Design review of the part built by this model. Coordinates are the model's own, in mm. A direction names the side the tool comes from. Round coordinates to 2 decimals unless told otherwise and drop trailing zeros. Loops run counter-clockwise (first coordinate to the right, second up) from the corner with the lowest first, then second, coordinate; pieces in that order, holes last. Notation, with made-up numbers: M -19.75,45 L 26.25,45 A30 cw 26.25,71 Z; hole C 18.5,-33 d10. An arc over 180 degrees is marked long. One line per item, written item: value. Start each with the question number.
Item 1: Clearance check with a flat-ended pin moving along its axis: pin 1 (1.3 mm diameter, centred on y = 3, z = -1, fed in from -X). State where the tip first meets the part, or that it passes through.
Item 2: We need section A-A (z = 1). Write out the cut boundary in (x, y), then the cut area to 3 significant figures.
Item 3: We need section D-D (x = 26). Write out the cut boundary in (y, z).
Item 4: For faces 1 (the flat face through (57.2, 0, -2)), 2 (the flat face through (4, -3.5, 1)), 3 (the flat face through (55.2, 0, -2)), list the 3-axis set-ups (+Z, -Z, +X, -X, +Y, -Y) from which the entire face can be reached by the end or side of a thin tool; tool diameter is ignored.
Item 5: We need section C-C (x = -33). Write out the cut boundary in (y, z), then the cut area to 3 significant figures.
Item 6: For line 1 along X through (y, z) = (-2.25, 1.25); line 2 along Z through (x, y) = (-1.5, -1.75); line 3 along Y through (x, z) = (48, -3.25), list the stretches that pass through material, from the lowest coordinate up.
Item 7: We need section B-B (y = 1.75). Write out the cut boundary in (x, z).
Item 8: Mouldability with a two-part tool opening along Z and no side actions: class faces 4 (the flat face through (0, -8.25, -2)), 5 (the flat face through (-1, 0, 0)), 6 (the flat face through (0, 0, -6.2)) as released by +Z, released by -Z, zero draft, split by the parting line, or undercut.
from build123d import *

# Parameters (mm, degrees)
F2_W     = 110.4
F2_H     = 12.5
F2_W_2   = 7
F2_H_2   = 7
F3_DEPTH = 2
F4_DEPTH = 2
F5_DEPTH = 2
F6_W     = 2
F6_H     = 4.2
F7_DEPTH = 110.4
F8_W     = 16.5
F8_H     = 8.2
F9_DEPTH = 2


with BuildPart() as f3:
    # F2 (on Top) → F3 (new body)
    with BuildSketch(Plane.XY):
        Rectangle(F2_W, F2_H)
        with Locations((-23.8, 0)):
            Rectangle(F2_W_2, F2_H_2, mode=Mode.SUBTRACT)
        with Locations((4.2, 0)):
            Rectangle(F2_W_2, F2_H_2, mode=Mode.SUBTRACT)
        with Locations((27.2, 0)):
            Rectangle(F2_W_2, F2_H_2, mode=Mode.SUBTRACT)
    extrude(amount=F3_DEPTH)

    # F4 (add): a face of the model
    f4_faces = [f3.faces().sort_by_distance(p)[0] for p in [
        (0, -6.25, 1),
    ]]
    extrude(f4_faces, amount=F4_DEPTH)

    # F5 (add): a face of the model
    f5_faces = [f3.faces().sort_by_distance(p)[0] for p in [
        (0, 6.25, 1),
    ]]
    extrude(f5_faces, amount=F5_DEPTH)

    # F6 (on face) → F7 (join)
    with BuildSketch(Plane(origin=(-55.2, 0, 0), x_dir=(0, -1, 0), z_dir=(-1, 0, 0))):
        with Locations((7.25, -2.1)):
            Rectangle(F6_W, F6_H)
        Polygon((-6.25, -4.2), (-8.25, -4.2), (-8.25, -6.2), (8.25, -6.2), (8.25, -4.2), (6.25, -4.2), align=None)
        with Locations((-7.25, -2.1)):
            Rectangle(F6_W, F6_H)
    extrude(amount=-F7_DEPTH)

    # F8 (on face) → F9 (join)
    with BuildSketch(Plane.YZ.offset(55.2)):
        with Locations((0, -2.1)):
            Rectangle(F8_W, F8_H)
    extrude(amount=F9_DEPTH)


solid = f3.part
A:
1. pin 1: x = 55.2
2. outline: M -55.2,-8.25 L 57.2,-8.25 L 57.2,8.25 L -55.2,8.25 Z; hole M -27.3,-3.5 L -20.3,-3.5 L -20.3,3.5 L -27.3,3.5 Z; hole M 0.7,-3.5 L 7.7,-3.5 L 7.7,3.5 L 0.7,3.5 Z; hole M 23.7,-3.5 L 30.7,-3.5 L 30.7,3.5 L 23.7,3.5 Z
2. area: 1,710 mm2
3. outline: M -8.25,-6.2 L 8.25,-6.2 L 8.25,2 L 3.5,2 L 3.5,0 L 6.25,0 L 6.25,-4.2 L -6.25,-4.2 L -6.25,0 L -3.5,0 L -3.5,2 L -8.25,2 Z
4. face 1: +Z, -Z, +X, +Y, -Y
4. face 2: +Z
4. face 3: -X
5. outline: M -8.25,-6.2 L 8.25,-6.2 L 8.25,2 L -8.25,2 Z; hole M -6.25,-4.2 L 6.25,-4.2 L 6.25,0 L -6.25,0 Z
5. area: 82.8 mm2
6. line 1: -55.2 to -27.3, -20.3 to 0.7, 7.7 to 23.7, 30.7 to 57.2
6. line 2: -6.2 to -4.2, 0 to 2
6. line 3: -8.25 to -6.25, 6.25 to 8.25
7. outline: M -55.2,-6.2 L 57.2,-6.2 L 57.2,2 L 30.7,2 L 30.7,0 L 55.2,0 L 55.2,-4.2 L -55.2,-4.2 Z; M -55.2,0 L -27.3,0 L -27.3,2 L -55.2,2 Z; M -20.3,0 L 0.7,0 L 0.7,2 L -20.3,2 Z; M 7.7,0 L 23.7,0 L 23.7,2 L 7.7,2 Z
8. face 4: zero draft
8. face 5: undercut
8. face 6: released by -Z
